Part model, mm, in its own coordinate system. A direction names the side the tool comes from. Round coordinates to 2 decimals unless told otherwise and drop trailing zeros. Write each loop counter-clockwise with the first axis right and the second up, starting at its lowest first coordinate (ties: lowest second). Pieces come first, ordered by that corner, then holes. Notation, with made-up numbers: M -39,-7.75 L -31,-7.75 A28 cw -31,15.25 Z; hole C 80.5,80.5 d11. An arc over 180 degrees is marked long. Use a Markdown table: item, result. Add a question column.
1) Slice it at D-D on x = -6.5. Write the cut outline in (y, z).
2) Slice it at A-A on y = 2.5. Write the cut outline in (x, z), plus the area to 3 significant figures.
3) Which spindle directions (+Z, -Z, +X, -X, +Y, -Y) get a long thin tool onto all of the face, cutting with end or side? Do faces 5 (the face through (-9.61, 1.52, -14.78)), 6 (the face through (0, 2, 15)). Say none if no direction does.
4) Drop flat-ended pins along their axis: P1, Ø6, axis at x = 0, z = 0, coming from the +Y side; P2, Ø4, axis at x = 3.5, z = 4.5, coming from the -Y side; P3, Ø3.5, axis at x = 1.5, z = 0.5, coming from the +Y side. Give the stop position or say it passes through.
5) Slice it at B-B on x = 0. Write the cut outline in (y, z).
6) Slice it at C-C on z = 2. Write the cut outline in (x, y), plus the area to 3 significant figures.
7) Wall check: probe 1 along Z at (x, y) = (0, 1.15); probe 2 along X at (y, z) = (1, 8); probe 3 along Y at (x, z) = (4.25, -1). Give the ranges that are in metal, low to high.
8) Two-plate mould, pull along X, no slides. Class faces 1 (the face through (-13.464, 5.406, -13.497)), 2 (the face through (4, 4, 0)), 3 (the face through (14.78, 3.76, -8.17)), 4 (the face through (-1.19, 5.01, 5.37)): released by +X, released by -X, zero draft, split by the parting line, or undercut.
```python
from build123d import *

# Parameters (mm, degrees)
SKETCH1_W                                           = 30
SKETCH1_H                                           = 30
BOSS_EXTRUDE1_DEPTH                                 = 6
CUT_EXTRUDE1_DEPTH                                  = 3
CUT_EXTRUDE2_DEPTH                                  = 22.424285286
FILLET1_R                                           = 3
CHAMFER1_SIZE                                       = 1.5
CBORE_FOR_M6_HEX_SOCKET_HEAD_CAP_SCREW1_D           = 6.6
CBORE_FOR_M6_HEX_SOCKET_HEAD_CAP_SCREW1_CBORE_D     = 11
CBORE_FOR_M6_HEX_SOCKET_HEAD_CAP_SCREW1_CBORE_DEPTH = 2


with BuildPart() as part:
    # Sketch1 → Boss-Extrude1 (new body)
    with BuildSketch(Plane(origin=(0, 0, 0), x_dir=(1, 0, 0), z_dir=(0, 1, 0))):
        Rectangle(SKETCH1_W, SKETCH1_H)
    extrude(amount=BOSS_EXTRUDE1_DEPTH)

    # Sketch2 → Cut-Extrude1 (cut)
    with BuildSketch(Plane.XZ):
        Polygon((15, 9.5), (-9.5, -15), (15, -15), align=None)
    extrude(amount=-CUT_EXTRUDE1_DEPTH, mode=Mode.SUBTRACT)

    # Sketch3 → Cut-Extrude2 (cut, through all)
    with BuildSketch(Plane.XZ.offset(-3)):
        Polygon((15, -8.282485579), (15, -15), (8.282485579, -15), align=None)
    extrude(amount=-CUT_EXTRUDE2_DEPTH, mode=Mode.SUBTRACT)

    # Fillet1
    fillet1_edges = [part.edges().sort_by_distance(p)[0] for p in [
        (15, 1.5, 9.5),
        (-9.5, 1.5, -15),
        (8.282485579, 4.5, -15),
        (15, 4.5, -8.282485579),
        (15, 3, 15),
        (-15, 3, 15),
        (-15, 3, -15),
    ]]
    fillet(fillet1_edges, radius=FILLET1_R)

    # Chamfer1
    chamfer1_edges = [part.edges().sort_by_distance(p)[0] for p in [
        (15, 6, 2.480077554),
        (-2.480077554, 6, -15),
        (0, 6, 15),
        (-15, 6, 0),
        (11.641242789, 6, -11.641242789),
        (14.121320344, 6, 14.121320344),
        (14.771638598, 6, -8.187895189),
        (8.187895189, 6, -14.771638598),
        (-14.121320344, 6, -14.121320344),
        (-14.121320344, 6, 14.121320344),
    ]]
    chamfer(chamfer1_edges, length=CHAMFER1_SIZE)

    # CBORE for M6 Hex Socket Head Cap Screw1 (through all)
    with Locations(Plane(origin=(0, 6, 0), x_dir=(1, 0, 0), z_dir=(0, 1, 0))):
        with Locations((0, 0)):
            CounterBoreHole(CBORE_FOR_M6_HEX_SOCKET_HEAD_CAP_SCREW1_D / 2, CBORE_FOR_M6_HEX_SOCKET_HEAD_CAP_SCREW1_CBORE_D / 2, CBORE_FOR_M6_HEX_SOCKET_HEAD_CAP_SCREW1_CBORE_DEPTH)


solid = part.part
```
Entries:
| question | item | result |
|---|---|---|
| 1 | outline | M 0,-12 L 3,-12 L 3,-15 L 4.5,-15 L 6,-13.5 L 6,13.5 L 4.5,15 L 0,15 Z |
| 2 | outline | M -15,-12 A3 ccw -12,-15 L -10.74,-15 A3 ccw -8.62,-14.12 L 14.12,8.62 A3 ccw 15,10.74 L 15,12 A3 ccw 12,15 L -12,15 A3 ccw -15,12 Z; hole C 0,0 d6.6 |
| 2 | area | 559 mm^2 |
| 3 | face 5 | -Z, +X, -Y |
| 3 | face 6 | +Z, +X, -X, +Y, -Y |
| 4 | P1 | passes through |
| 4 | P2 | stops at y = 0 |
| 4 | P3 | stops at y = 4 |
| 5 | outline | M 0,-5.5 L 3,-5.5 L 3,-15 L 4.5,-15 L 6,-13.5 L 6,-5.5 L 4,-5.5 L 4,-3.3 L 0,-3.3 Z; M 0,3.3 L 4,3.3 L 4,5.5 L 6,5.5 L 6,13.5 L 4.5,15 L 0,15 Z |
| 6 | outline | M -15,0 L -2.62,0 L -2.62,4 L -5.12,4 L -5.12,6 L -13.5,6 L -15,4.5 Z; M 2.62,0 L 7.5,0 L 7.5,3 L 15,3 L 15,4.5 L 13.5,6 L 5.12,6 L 5.12,4 L 2.62,4 Z |
| 6 | area | 114 mm^2 |
| 7 | probe 1 | z = -5.5 to -3.3, 3.3 to 15 |
| 7 | probe 2 | x = -15 to 13.5 |
| 7 | probe 3 | y = 0 to 4 |
| 8 | face 1 | released by -X |
| 8 | face 2 | undercut |
| 8 | face 3 | released by +X |
| 8 | face 4 | undercut |
